```python
from build123d import *

# Parameters (mm, degrees)
SKETCH_W                   = 30
SKETCH_H                   = 15
PAD_DEPTH                  = 3.5
POCKET_DEPTH               = 15.001
LINEARPATTERN_COUNT        = 2
LINEARPATTERN_PITCH        = 15
SKETCH003_W                = 4
SKETCH003_H                = 2
PAD001_DEPTH               = 2.5
SKETCH003_MIRRORED_2_W     = 4
SKETCH003_MIRRORED_2_H     = 2
PAD001_MIRRORED_2_DEPTH    = 2.5
SKETCH004_W                = 30
SKETCH004_H                = 15
SKETCH004_W_2              = 28
SKETCH004_H_2              = 13
PAD002_DEPTH               = 9.5
SKETCH005_W                = 1
SKETCH005_H                = 1
PAD003_DEPTH               = 2
SKETCH005_MIRRORED002_2_W  = 1
SKETCH005_MIRRORED002_2_H  = 1
PAD003_MIRRORED002_2_DEPTH = 2
SKETCH006_W                = 4
SKETCH006_H                = 1
PAD004_DEPTH               = 1
CHAMFER_SIZE               = 0.5


with BuildPart() as part:
    # Sketch → Pad (new body)
    with BuildSketch(Plane.XY):
        Rectangle(SKETCH_W, SKETCH_H)
    extrude(amount=PAD_DEPTH)

    # Sketch002 (on Face3 of Pad) → Pocket (cut, through all)
    with BuildSketch(Plane.XZ.offset(7.5)):
        with BuildLine():
            Line((-9, 0.722949), (-9, 0))
            Line((-9, 0), (-6, 0))
            Line((-6, 0.722949), (-6, 0))
            ThreePointArc((-6, 0.722949), (-5.37226, 1.668412), (-5.285841, 2.8))
            Line((-9.714159, 2.8), (-5.285841, 2.8))
            ThreePointArc((-9.714159, 2.8), (-9.62774, 1.668412), (-9, 0.722949))
        make_face()
    pocket = extrude(amount=-POCKET_DEPTH, mode=Mode.SUBTRACT)

    # LinearPattern: Pocket ×2
    with Locations(*[(i * LINEARPATTERN_PITCH, 0, 0) for i in range(1, LINEARPATTERN_COUNT)]):
        add(pocket, mode=Mode.SUBTRACT)

    # Sketch003 (on Face16 of LinearPattern) → Pad001 (join)
    with BuildSketch(Plane.XY.offset(3.5)):
        with Locations((-12, 5.5)):
            Rectangle(SKETCH003_W, SKETCH003_H)
    pad001 = extrude(amount=PAD001_DEPTH)

    # Sketch003 Mirrored 2 → Pad001 Mirrored 2 (add)
    with BuildSketch(Plane(origin=(0, 0, 3.5), x_dir=(-1, 0, 0), z_dir=(0, 0, -1))):
        with Locations((-12, 5.5)):
            Rectangle(SKETCH003_MIRRORED_2_W, SKETCH003_MIRRORED_2_H)
    pad001_mirrored_2 = extrude(amount=-PAD001_MIRRORED_2_DEPTH)

    # Mirrored001: Pad001, Pad001 Mirrored 2 across XZ
    add(pad001.mirror(Plane.XZ))
    add(pad001_mirrored_2.mirror(Plane.XZ))

    # Sketch004 (on Face16 of MultiTransform) → Pad002 (join)
    with BuildSketch(Plane.XY.offset(3.5)):
        Rectangle(SKETCH004_W, SKETCH004_H)
        Rectangle(SKETCH004_W_2, SKETCH004_H_2, mode=Mode.SUBTRACT)
    extrude(amount=PAD002_DEPTH)

    # Sketch005 (on Face31 of Pad002) → Pad003 (join)
    with BuildSketch(Plane.XY.offset(6)):
        with Locations((-10.5, 6)):
            Rectangle(SKETCH005_W, SKETCH005_H)
        with Locations((-13.5, 5)):
            Rectangle(SKETCH005_W, SKETCH005_H)
    pad003 = extrude(amount=PAD003_DEPTH)

    # Sketch005 Mirrored002 2 → Pad003 Mirrored002 2 (add)
    with BuildSketch(Plane(origin=(0, 0, 6), x_dir=(-1, 0, 0), z_dir=(0, 0, -1))):
        with Locations((-10.5, 6)):
            Rectangle(SKETCH005_MIRRORED002_2_W, SKETCH005_MIRRORED002_2_H)
        with Locations((-13.5, 5)):
            Rectangle(SKETCH005_MIRRORED002_2_W, SKETCH005_MIRRORED002_2_H)
    pad003_mirrored002_2 = extrude(amount=-PAD003_MIRRORED002_2_DEPTH)

    # Mirrored003: Pad003, Pad003 Mirrored002 2 across XZ
    add(pad003.mirror(Plane.XZ))
    add(pad003_mirrored002_2.mirror(Plane.XZ))

    # Sketch006 (on Face26 of MultiTransform001) → Pad004 (join)
    with BuildSketch(Plane.XZ.offset(-6.5)):
        with Locations((0, 12.5)):
            Rectangle(SKETCH006_W, SKETCH006_H)
    pad004 = extrude(amount=PAD004_DEPTH)

    # Mirrored004: Pad004 across XZ
    add(pad004.mirror(Plane.XZ))

    # Chamfer
    chamfer_edges = [part.edges().sort_by_distance(p)[0] for p in [
        (0, 5.5, 13),
        (0, -5.5, 13),
    ]]
    chamfer(chamfer_edges, length=CHAMFER_SIZE)


solid = part.part
```
Can you work these out from the model? Positions are in its coordinate system, mm. A direction names the side the tool comes from. Coordinates: 2 decimals unless noted, no trailing zeros. Loops run counter-clockwise (first coordinate to the right, second up) from the corner with the lowest first, then second, coordinate; pieces in that order, holes last.
1) Imagine slicing it at B-B on x = 11.5. List the corners of the cut face in (y, z) for me, plus the area to 3 significant figures.
2) I need wall thicknesses on probe 1 along Y at (x, z) = (-10, 12); probe 2 along X at (y, z) = (-2, 5.25); probe 3 along X at (y, z) = (-5.75, 5.75). Which ranges of each line are inside material? Lowest first, please.
3) Imagine slicing it at A-A on z = 9.5. List the corners of the cut face in (x, y) for me, plus the area to 3 significant figures.
4) Thinking about a two-plate mould opening in Z: for faces 1 (the cylindrical face through (5.37, -0.11, 1.68)), 2 (the flat face through (13.5, -5, 8)), 3 (the flat face through (-12, 4.5, 5)), 4 (the flat face through (0, -6, 12)), which applies, pulls with the +Z half, pulls with the -Z half, needs draft (parallel to the pull), parting line crosses it, or undercut?
5) Imagine slicing it at D-D on x = 3.25. List the corners of the cut face in (y, z) for me.
6) Imagine slicing it at C-C on y = 3.75. List the corners of the cut face in (x, z) for me, plus the area to 3 significant figures.
7) For pin 1 (8 mm diameter, centred on x = -3, y = -3.5, fed in from +Z), with a flat end and sliding along its axis, tell me the tip position at first contact or that it passes through.
8) Which directions (+Z, -Z, +X, -X, +Y, -Y) give clear straight access to the entire face, cutting with the end or side of a thin tool? Please do faces 5 (the flat face through (15, 0, 6)), 6 (the flat face through (7, 0, 2.8)), 7 (the flat face through (-10, 6, 5)).
Completed:
1. outline: (-7.5, 0) - (7.5, 0) - (7.5, 13) - (6.5, 13) - (6.5, 6) - (4.5, 6) - (4.5, 3.5) - (-4.5, 3.5) - (-4.5, 6) - (-6.5, 6) - (-6.5, 13) - (-7.5, 13) - close
1. area: 81.5 mm2
2. probe 1: y = -7.5 to -6.5, 6.5 to 7.5
2. probe 2: x = -15 to -14, 14 to 15
2. probe 3: x = -15 to -10, 10 to 15
3. outline: (-15, -7.5) - (15, -7.5) - (15, 7.5) - (-15, 7.5) - close; hole (-14, -6.5) - (14, -6.5) - (14, 6.5) - (-14, 6.5) - close
3. area: 86.0 mm2
4. face 1: undercut
4. face 2: pulls with the +Z half
4. face 3: needs draft
4. face 4: undercut
5. outline: (-7.5, 0) - (7.5, 0) - (7.5, 13) - (6.5, 13) - (6.5, 3.5) - (-6.5, 3.5) - (-6.5, 13) - (-7.5, 13) - close
6. outline: (-15, 0) - (-9, 0) - (-9, 0.72) arc R2.25 cw to (-9.71, 2.8) - (-5.29, 2.8) arc R2.25 cw to (-6, 0.72) - (-6, 0) - (6, 0) - (6, 0.72) arc R2.25 cw to (5.29, 2.8) - (9.71, 2.8) arc R2.25 cw to (9, 0.72) - (9, 0) - (15, 0) - (15, 13) - (14, 13) - (14, 3.5) - (-14, 3.5) - (-14, 13) - (-15, 13) - close
6. area: 103 mm2
7. pin 1: stops at z = 13
8. face 5: +Z, -Z, +X, +Y, -Y
8. face 6: +Y, -Y
8. face 7: +Z
